Autodesk Inventor part; units mm, degrees
ref_plane "YZ Plane" through (0, 0, 0) normal (1, 0, 0) x (0, 1, 0)
ref_plane "XZ Plane" through (0, 0, 0) normal (0, 1, 0) x (-1, 0, 0)
ref_plane "XY Plane" through (0, 0, 0) normal (0, 0, 1) x (1, 0, 0)
sketch "Skizze2" plane through (0, 0, 0) normal (0, 0, 1) x (1, 0, 0)
  line L0 (-775, 525) -> (575, 525)
  line L1 (975, 125) -> (975, -25)
  line L2 (575, -425) -> (-775, -425)
  line L3 (-975, -225) -> (-975, 325)
  arc A0 (975, 125) -> (575, 525) centre (575, 125) ccw
  arc A1 (575, -425) -> (975, -25) centre (575, -25) ccw
  arc A2 (-775, 525) -> (-975, 325) centre (-775, 325) ccw
  arc A3 (-975, -225) -> (-775, -425) centre (-775, -225) ccw
  circle A4 centre (0, 50) radius 360
  point P0 (0, 0)
  point P1 (975, -425)
  point P2 (975, 525)
  point P3 (-975, -425)
  dimension "d0" = 950
  dimension "d1" = 1950
  dimension "d2" = 400
  dimension "d3" = 200
  dimension "d4" = 720
  dimension "d5" = 975
  dimension "d6" = 475
extrude "Extrusion1" add sketch "Skizze2" against normal blind 100
sketch "Skizze3" plane through (-775, -425, 0) normal (0, -1, 0) x (1, 0, 0)
  line L0 (1750, 0) -> (1350, 0)
  line L1 (1350, -100) -> (1750, -100)
  line L2 (1350, 0) -> (1750, 0)
  line L3 (1750, 0) -> (1750, -100)
  line L4 (1750, -100) -> (1350, -100)
  line L5 (1350, -100) -> (1350, 0)
  line L6 (1750, -100) -> (1679.3683, -100)
  line L7 (1670, -35) -> (1750, -35)
  line L8 (1750, -35) -> (1750, -100)
  ellipse E0 centre (1679.3683, -100) end of major axis (1670, -35) minor radius 127.378 (1670, -35) -> (1555.4261, -100) ccw
  point P0 (775, 0)
  dimension "d11" = 65
  dimension "d12" = 80
extrude "Extrusion2" cut sketch "Skizze3" against normal through all contours L3 L1 E0 L7
sketch "Skizze4" plane through (0, 0, -100) normal (0, 0, -1) x (-1, 0, 0)
  line L0 (975, -410) -> (-975, -410)
  line L1 (-975, -410) -> (-975, -315)
  line L2 (-975, -315) -> (975, -315)
  line L3 (975, -315) -> (975, -410)
  line L4 (975, -225) -> (975, 325)
  line L5 (-975, -25) -> (-975, 125)
  line L6 (-575, -425) -> (775, -425)
  line L7 (975, 415) -> (-975, 415)
  line L8 (-975, 415) -> (-975, 510)
  line L9 (-975, 510) -> (975, 510)
  line L10 (975, 510) -> (975, 415)
  line L11 (775, 525) -> (-575, 525)
  point P0 (0, 0)
  dimension "d15" = 95
  dimension "d16" = 0
  dimension "d17" = 0
  dimension "d19" = 15
  dimension "d20" = 95
  dimension "d21" = 0
  dimension "d22" = 0
  dimension "d23" = 15
extrude "Extrusion3" cut sketch "Skizze4" against normal blind 20
sketch "Skizze5" plane through (0, 0, -80) normal (0, 0, -1) x (-1, 0, 0)
  line L0 (953.6057, 415) -> (-793.3777, 415)
  line L1 (953.6057, 415) -> (-793.3777, 415)
  line L2 (-793.3777, 415) -> (-793.3777, 460.1286)
  line L3 (-793.3777, 415) -> (-793.3777, 460.1286)
  line L4 (-683.5127, 510) -> (850.9934, 510)
  line L5 (850.9934, 510) -> (-683.5127, 510)
  arc A0 (-683.5127, 510) -> (-793.3777, 460.1286) centre (-575, 125) ccw
  arc A1 (953.6057, 415) -> (850.9934, 510) centre (775, 325) ccw
  point P0 (0, 0)
sketch "Skizze6" plane through (-953.6057, 415, -100) normal (0, 1, 0) x (1, 0, 0)
  ellipse E0 centre (1857.974, 0) end of major axis (1731.8988, 18.1709) minor radius 65.6716 (1734.0318, 0) -> (1746.9834, -20) ccw
  arc A0 (1734.0318, 0) -> (1746.9834, -20) centre (1792.2814, 23.5278) ccw
  line L0 (1734.0318, 0) -> (1856.261, 0)
  line L1 (1856.261, 0) -> (1856.261, -20)
  line L2 (1856.261, -20) -> (1746.9834, -20)
  point P0 (953.6057, -100)
properties part number "XPS" material "Polystyrol"
Input: part model. Units: mm. Frame: model coordinates. A direction names the side the tool comes from. Round coordinates to 2 decimals unless told otherwise and drop trailing zeros. Loops run counter-clockwise (first coordinate to the right, second up) from the corner with the lowest first, then second, coordinate; pieces in that order, holes last. Notation, with made-up numbers: (-13, 39) -> (25, 39) arc R16 cw to (25, 69) -> close; hole circle Ø1 at (-29, 7.25). An arc over 180 degrees is marked (long way). Write each question's results on one line, items separated by ' | '.
1. Mould query, pull axis Y, two halves, no side actions, for faces 4 (the face through (800.814, -355.164, -38.189)), 5 (the face through (-68, 463, -80)), 6 (the face through (-305, 298, -100)), 7 (the face through (166.12, -269.38, -49.3)). Classes: +Y half, -Y half, draft (parallel to the pull), parting line (faces both ways), or undercut.
Geometry results:
face 4: -Y half | face 5: undercut | face 6: draft | face 7: undercut
2. Section A-A (x = 0). Return loops of the section in (y, z), and give its area (3 significant figures).
Geometry results:
outline: (-425, -100) -> (-410, -100) -> (-410, -80) -> (-315, -80) -> (-315, -100) -> (-310, -100) -> (-310, 0) -> (-425, 0) -> close; (410, -100) -> (415, -100) -> (415, -80) -> (510, -80) -> (510, -100) -> (525, -100) -> (525, 0) -> (410, 0) -> close | area: 19,200 mm2
3. Set-up query: faces 1 (the face through (-975, 46, -49)), 2 (the face through (926, 46, -35)), 3 (the face through (-68, -362, -80)). Return all of +Z, -Z, +X, -X, +Y, -Y with unobstructed straight access to the full face (end or side cutting, diameter ignored); none if empty.
Geometry results:
face 1: +Z, -Z, -X, +Y, -Y | face 2: -Z, +X, +Y, -Y | face 3: -Z, +X, -X
4. Section D-D (x = 252). Return loops of the section in (y, z).
Geometry results:
outline: (-425, -100) -> (-410, -100) -> (-410, -80) -> (-315, -80) -> (-315, -100) -> (-207.09, -100) -> (-207.09, 0) -> (-425, 0) -> close; (307.09, -100) -> (415, -100) -> (415, -80) -> (510, -80) -> (510, -100) -> (525, -100) -> (525, 0) -> (307.09, 0) -> close
5. First-contact query: P1, Ø1.5, axis at y = 198, z = -21, coming from the +X side; P2, Ø12, axis at x = 340.5, y = -33.5, coming from the +Z side; P3, Ø4, axis at y = 260.5, z = -12, coming from the +X side. Flat tips, straight axial feed; report the tip coordinate or a pass-through.
Geometry results:
P1: x = 968.42 | P2: through | P3: x = 952.06
6. Ray query, line 1 (Y direction, x = 0, z = -72); line 2 (Y direction, x = -125.5, z = -16); line 3 (X direction, y = 112.5, z = -17.5). Return the intervals inside material, ascending. Write a range as from..to.
Geometry results:
line 1: -425..-310, 410..525 | line 2: -425..-287.42, 387.42..525 | line 3: -975..-354.53, 354.53..975
7. Section C-C (x = 476). Return loops of the section in (y, z).
Geometry results:
outline: (-425, -100) -> (-410, -100) -> (-410, -80) -> (-315, -80) -> (-315, -100) -> (415, -100) -> (415, -80) -> (510, -80) -> (510, -100) -> (525, -100) -> (525, 0) -> (-425, 0) -> close
8. Section B-B (z = -17). Return loops of the section in (x, y).
Geometry results:
outline: (-975, -225) arc R200 ccw to (-775, -425) -> (575, -425) arc R400 ccw to (975, -25) -> (975, 125) arc R400 ccw to (575, 525) -> (-775, 525) arc R200 ccw to (-975, 325) -> close; hole circle Ø720 at (0, 50)
